```python
from build123d import *

# Parameters (mm, degrees)
SKETCH016_W     = 8
SKETCH016_H     = 18
SKETCH016_W_2   = 1.2
SKETCH016_H_2   = 4.1
PAD011_DEPTH    = 10
SKETCH017_R     = 2.5
POCKET009_DEPTH = 8
FILLET001_R     = 1
CHAMFER001_SIZE = 0.3
CHAMFER002_SIZE = 0.3


with BuildPart() as part:
    # Sketch016 → Pad011 (new body)
    with BuildSketch(Plane.XY):
        with Locations((0, 3.95)):
            Rectangle(SKETCH016_W, SKETCH016_H)
        Rectangle(SKETCH016_W_2, SKETCH016_H_2, mode=Mode.SUBTRACT)
    extrude(amount=PAD011_DEPTH)

    # Sketch017 (on Face1 of Pad011) → Pocket009 (cut)
    with BuildSketch(Plane(origin=(0, 12.95, 0), x_dir=(-1, 0, 0), z_dir=(0, 1, 0))):
        with Locations((0, 5)):
            Circle(SKETCH017_R)
    extrude(amount=-POCKET009_DEPTH, mode=Mode.SUBTRACT)

    # Fillet001
    fillet001_edges = [part.edges().sort_by_distance(p)[0] for p in [
        (4, 3.95, 0),
        (4, 3.95, 10),
        (-4, 3.95, 10),
        (-4, 3.95, 0),
    ]]
    fillet(fillet001_edges, radius=FILLET001_R)

    # Chamfer001
    chamfer001_edges = [part.edges().sort_by_distance(p)[0] for p in [
        (0, -2.05, 0),
        (0.6, 0, 0),
        (0, 2.05, 0),
        (-0.6, 0, 0),
    ]]
    chamfer(chamfer001_edges, length=CHAMFER001_SIZE)

    # Chamfer002
    chamfer002_edges = [part.edges().sort_by_distance(p)[0] for p in [
        (-0.6, 0, 10),
        (0, -2.05, 10),
        (0.6, 0, 10),
        (0, 2.05, 10),
    ]]
    chamfer(chamfer002_edges, length=CHAMFER002_SIZE)


solid = part.part
```
Check sheet for the modelled part. Datum: model origin and axes. Units: mm. A direction names the side the tool comes from. Round coordinates to 2 decimals unless told otherwise and drop trailing zeros. Write each loop counter-clockwise with the first axis right and the second up, starting at its lowest first coordinate (ties: lowest second). Pieces come first, ordered by that corner, then holes. Notation, with made-up numbers: (51.5, 16) -> (82.5, 16) arc R34 ccw to (82.5, 53) -> close; hole circle Ø5 at (46.5, 48). An arc over 180 degrees is marked (long way). One line per question, with ' | ' between items. Start each with the question number.
1. Sectioned sample at D-D, the plane x = -1.75. Record the cut outline in (y, z).
2. Set-up check for faces 1 (the face through (0, 4.95, 5)), 2 (the face through (0.6, 0, 5)), 3 (the face through (0, 4, 10)): record each of +Z, -Z, +X, -X, +Y, -Y from which the full face is reachable in a straight line by a thin tool's end or side.
3. Sectioned sample at A-A, the plane x = 0. Record the cut outline in (y, z), then the cut area to 3 significant figures.
4. Release check for a two-part mould opening along X. For faces 4 (the face through (-4, 4, 5)), 5 (the face through (3.699, 4.076, 0.285)), 6 (the face through (0, -2.05, 5)) record: +X half, -X half, draft (parallel to the pull), parting line (faces both ways), or undercut.
5. Sectioned sample at C-C, the plane z = 6.5. Record the cut outline in (x, y), then the cut area to 3 significant figures.
6. Scan lines: line 1 along Y through (x, z) = (0.25, 5); line 2 along Y through (x, z) = (-0.5, 8); line 3 along Z through (x, y) = (0, 7). Record each from-to range of solid material in increasing order. Write a range as from..to.
7. Sectioned sample at B-B, the plane y = -0.75. Record the cut outline in (x, z).
8. Depth check by flat-ended pin: pin 1 (2.5 mm diameter, centred on x = 0.5, z = 6, fed in from +Y). Enter the tip coordinate at first touch or a pass-through.
Taken from the geometry:
1) outline: (-5.05, 0) -> (12.95, 0) -> (12.95, 3.21) -> (4.95, 3.21) -> (4.95, 6.79) -> (12.95, 6.79) -> (12.95, 10) -> (-5.05, 10) -> close
2) face 1: +Y | face 2: +Z, -Z | face 3: +Z, +X, -X, +Y, -Y
3) outline: (-5.05, 0) -> (-2.35, 0) -> (-2.05, 0.3) -> (-2.05, 9.7) -> (-2.35, 10) -> (-5.05, 10) -> close; (2.05, 0.3) -> (2.35, 0) -> (12.95, 0) -> (12.95, 2.5) -> (4.95, 2.5) -> (4.95, 7.5) -> (12.95, 7.5) -> (12.95, 10) -> (2.35, 10) -> (2.05, 9.7) -> close | area: 98.8 mm^2
4) face 4: -X half | face 5: +X half | face 6: undercut
5) outline: (-4, -5.05) -> (4, -5.05) -> (4, 12.95) -> (2, 12.95) -> (2, 4.95) -> (-2, 4.95) -> (-2, 12.95) -> (-4, 12.95) -> close; hole (-0.6, -2.05) -> (0.6, -2.05) -> (0.6, 2.05) -> (-0.6, 2.05) -> close | area: 107 mm^2
6) line 1: y = -5.05..-2.05, 2.05..4.95 | line 2: y = -5.05..-2.05, 2.05..12.95 | line 3: z = 0..2.5, 7.5..10
7) outline: (-4, 1) arc R1 ccw to (-3, 0) -> (-0.9, 0) -> (-0.6, 0.3) -> (-0.6, 9.7) -> (-0.9, 10) -> (-3, 10) arc R1 ccw to (-4, 9) -> close; (0.6, 0.3) -> (0.9, 0) -> (3, 0) arc R1 ccw to (4, 1) -> (4, 9) arc R1 ccw to (3, 10) -> (0.9, 10) -> (0.6, 9.7) -> close
8) pin 1: stops at y = 4.95
